Read the model definition and answer for the solid it produces. Units are mm, in the model's axes. Face numbers are marked on the shaded views. A direction names the side the tool comes from. Give positions to 0.01 mm unless a question says otherwise; leave off trailing zeros. Order: outer loops, then holes, each group sorted by start corner. A loop starts at its lowest first (then second) coordinate and runs counter-clockwise, first axis right, second up.
Item 1: The mould has two halves that part along Y. Classify the marked faces 1, 2 and 3: +Y half, -Y half, draft (parallel to the pull), parting line (faces both ways), or undercut.
Item 2: Find the intervals of material crossed by line 1 along X through (y, z) = (-4.25, 1); line 2 along Y through (x, z) = (-4.25, 4.75); line 3 along Z through (x, y) = (-2.75, 1.5), in increasing order.
Item 3: Which of the six approach directions +Z, -Z, +X, -X, +Y, -Y give full straight-line access (tool end or side, diameter ignored) to the marked faces 4 and 5?
Item 4: A cutting plane is placed at A-A (y = 4). Write down the section's boundary in (x, z), plus the area to 3 significant figures.
Item 5: A cutting plane is placed at B-B (x = -3). Write down the section's boundary in (y, z).
Item 6: A cutting plane is placed at C-C (y = 0). Write down the section's boundary in (x, z), plus the area to 3 significant figures.
Item 7: Given pin 1 Ø3 at (y, z) = (2, 6) entering from +X (3 decimals); pin 2 Ø0.8 at (y, z) = (3, 7.5) entering from -X (3 decimals); pin 3 Ø0.5 at (y, z) = (1.5, 7.5) entering from +X, each flat-ended and moving along its own axis, determine where each tip first touches the part or whether it passes through.
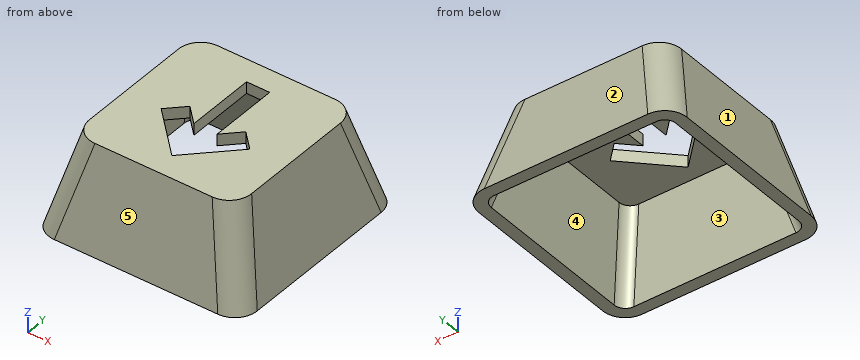
from build123d import *

# Parameters (mm, degrees)
SKETCH_W             = 18
SKETCH_H             = 18
PAD_DEPTH            = 8
POCKET_DEPTH         = 18.001
POCKET001_DEPTH      = 9.001
POCKET001_DEPTH_BACK = 9.001
FILLET_R             = 2
THICKNESS_T          = -1
POCKET002_DEPTH      = 5.01


with BuildPart() as part:
    # Sketch → Pad (new body)
    with BuildSketch(Plane.XY):
        Rectangle(SKETCH_W, SKETCH_H)
    extrude(amount=PAD_DEPTH)

    # Sketch001 (on Face1 of Pad) → Pocket (cut, through all)
    with BuildSketch(Plane.XZ.offset(9)):
        Polygon((-9, 8), (-9, 0), (-7, 8), align=None)
        Polygon((9, 8), (9, 0), (7, 8), align=None)
    extrude(amount=-POCKET_DEPTH, mode=Mode.SUBTRACT)

    # Sketch002 → Pocket001 (cut, two sides)
    with BuildSketch(Plane.YZ) as pocket001_sk:
        Polygon((-9, 8), (-7, 8), (-9, 0), align=None)
        Polygon((9, 8), (7, 8), (9, 0), align=None)
    extrude(amount=-POCKET001_DEPTH, mode=Mode.SUBTRACT)
    extrude(pocket001_sk.sketch, amount=POCKET001_DEPTH_BACK, mode=Mode.SUBTRACT)

    # Fillet
    fillet_edges = [part.edges().sort_by_distance(p)[0] for p in [
        (-8, 8, 4),
        (-8, -8, 4),
        (8, -8, 4),
        (8, 8, 4),
    ]]
    fillet(fillet_edges, radius=FILLET_R)

    # Thickness
    thickness_openings = [part.faces().sort_by_distance(p)[0] for p in [
        (0, 0, 0),
    ]]
    offset(amount=THICKNESS_T, openings=thickness_openings, kind=Kind.INTERSECTION)

    # Sketch003 (on Face9 of Thickness) → Pocket002 (cut)
    with BuildSketch(Plane.XY.offset(8)):
        Polygon((-1, 4.914214), (1, 4.914214), (1, -1.085786), (2.414214, 0.328427), (3.828427, -1.085786), (0, -4.914214), (-3.828427, -1.085786), (-2.414214, 0.328427), (-1, -1.085786), align=None)
    extrude(amount=-POCKET002_DEPTH, mode=Mode.SUBTRACT)


solid = part.part
Response values:
1. face 1: draft
1. face 2: +Y half
1. face 3: undercut
2. line 1: x = -8.75 to -7.72, 7.72 to 8.75
2. line 2: y = -7.81 to -6.78, 6.78 to 7.81
2. line 3: z = 7 to 8
3. face 4: -Z
3. face 5: +Z, +X, -X, -Y
4. outline: (-9, 0) - (-7.97, 0) - (-6.22, 7) - (-1, 7) - (-1, 8) - (-7, 8) - close; (1, 7) - (6.22, 7) - (7.97, 0) - (9, 0) - (7, 8) - (1, 8) - close
4. area: 26.7 mm2
5. outline: (-9, 0) - (-7.97, 0) - (-6.22, 7) - (-1.91, 7) - (-1.91, 8) - (-7, 8) - close; (-0.26, 7) - (6.22, 7) - (7.97, 0) - (9, 0) - (7, 8) - (-0.26, 8) - close
6. outline: (-9, 0) - (-7.97, 0) - (-6.22, 7) - (-2.74, 7) - (-2.74, 8) - (-7, 8) - close; (-2.09, 7) - (-1, 7) - (-1, 8) - (-2.09, 8) - close; (1, 7) - (2.09, 7) - (2.09, 8) - (1, 8) - close; (2.74, 7) - (6.22, 7) - (7.97, 0) - (9, 0) - (7, 8) - (2.74, 8) - close
6. area: 25.4 mm2
7. pin 1: stops at x = 7.875
7. pin 2: stops at x = -7.225
7. pin 3: stops at x = 7.19
